Autodesk Inventor part; units mm, degrees
ref_plane "YZ Plane" through (0, 0, 0) normal (1, 0, 0) x (0, 1, 0)
ref_plane "XZ Plane" through (0, 0, 0) normal (0, 1, 0) x (-1, 0, 0)
ref_plane "XY Plane" through (0, 0, 0) normal (0, 0, 1) x (1, 0, 0)
sketch "Sketch1" plane through (0, 0, 0) normal (0, 1, 0) x (-1, 0, 0)
  line L0 (0, 0) -> (-269.875, 0)
  line L1 (-269.875, 0) -> (-269.875, -157.1625)
  line L2 (-269.875, -157.1625) -> (0, -157.1625)
  line L3 (0, -157.1625) -> (0, 0)
  circle A0 centre (-257.175, -148.2725) radius 2.7559
  circle A1 centre (-257.175, -8.89) radius 2.7559
  circle A2 centre (-12.7, -8.89) radius 2.7559
  circle A3 centre (-257.175, -131.1275) radius 2.7559
  circle A4 centre (-257.175, -26.035) radius 2.7559
  circle A5 centre (-12.7, -148.2725) radius 2.7559
  circle A6 centre (-12.7, -131.1275) radius 2.7559
  circle A7 centre (-12.7, -26.035) radius 2.7559
  circle A8 centre (-244.475, -62.5475) radius 4.6609
  line L4 (-242.5434, -66.7893) -> (-246.4066, -66.7893)
  line L5 (-254, -66.7893) -> (-254, -58.3057) construction
  line L6 (-246.4066, -58.3057) -> (-242.5434, -58.3057)
  line L7 (-236.5375, -58.3057) -> (-236.5375, -66.7893) construction
  dimension "d0" = 157.1625
  dimension "d1" = 269.875
  dimension "d2" = 12.7
  dimension "d3" = 8.89
  dimension "d6" = 8.89
  dimension "d7" = 12.7
  dimension "d8" = 12.7
  dimension "d9" = 8.89
  dimension "d11" = 5.5118
  dimension "d12" = 5.5118
  dimension "d13" = 5.5118
  dimension "d15" = 17.145
  dimension "d16" = 12.7
  dimension "d17" = 5.5118
  dimension "d18" = 5.5118
  dimension "d19" = 12.7
  dimension "d20" = 17.145
  dimension "d21" = 12.7
  dimension "d22" = 8.89
  dimension "d23" = 5.5118
  dimension "d24" = 17.145
  dimension "d25" = 12.7
  dimension "d26" = 5.5118
  dimension "d27" = 12.7
  dimension "d28" = 17.145
  dimension "d29" = 5.5118
  dimension "d32" = 25.4
  dimension "d33" = 9.3218
  dimension "d34" = 4.2418
  dimension "d35" = 4.2418
  dimension "d36" = 17.4625
  dimension "d37" = 15.875
  dimension "d38" = 94.615
extrude "Extrusion2" add sketch "Sketch1" along normal blind 5.7658 contours L3 L2 L1 L0 | L6 A8 | A8 L4
properties part number "2023 1 17 Computer Box Door" material "Polycarbonate, Clear"
Check sheet for the modelled part. Datum: model origin and axes. Units: mm. A direction names the side the tool comes from. Coordinates: 2 decimals unless noted, no trailing zeros. Loops run counter-clockwise (first coordinate to the right, second up) from the corner with the lowest first, then second, coordinate; pieces in that order, holes last. Notation, with made-up numbers: (5.5, 23) -> (41.5, 23) arc R22 cw to (41.5, 47) -> close; hole circle Ø6 at (39, 53.5). An arc over 180 degrees is marked (long way). Write item = value, one per line. Start each with the question number.
1. Tool access check on faces 1 (the flat face through (137, 0, -77)), 2 (the cylindrical face through (239.815, 2.843, -62.473)). Record the directions out of +Z, -Z, +X, -X, +Y, -Y that give a thin tool (end or side, any length) a straight path to the whole face; none if there is none.
2. Draft check along X on faces 3 (the cylindrical face through (13.059, 2.843, -11.622)), 4 (the flat face through (269.875, 3, -77)), 5 (the flat face through (137, 5.766, -77)). Enter one of: released by +X, released by -X, zero draft, split by the parting line, or undercut.
3. Section check A-A on x = 12.7. Record the cut outline in (y, z).
4. Material ranges on line 1 (Z direction, x = 12.7, y = 3.15), recorded low to high.
5. Section check B-B on z = -8.89. Record the cut outline in (x, y) (3 decimals), then the cut area to 3 significant figures.
Responses:
q1.face_1 = +Z, -Z, +X, -X, -Y
q1.face_2 = +Y, -Y
q2.face_3 = undercut
q2.face_4 = released by +X
q2.face_5 = zero draft
q3.outline = (0, -157.16) -> (5.77, -157.16) -> (5.77, -151.03) -> (0, -151.03) -> close; (0, -145.52) -> (5.77, -145.52) -> (5.77, -133.88) -> (0, -133.88) -> close; (0, -128.37) -> (5.77, -128.37) -> (5.77, -28.79) -> (0, -28.79) -> close; (0, -23.28) -> (5.77, -23.28) -> (5.77, -11.65) -> (0, -11.65) -> close; (0, -6.13) -> (5.77, -6.13) -> (5.77, 0) -> (0, 0) -> close
q4.line_1 = -157.16 to -151.03, -145.52 to -133.88, -128.37 to -28.79, -23.28 to -11.65, -6.13 to 0
q5.outline = (0, 0) -> (9.944, 0) -> (9.944, 5.766) -> (0, 5.766) -> close; (15.456, 0) -> (254.419, 0) -> (254.419, 5.766) -> (15.456, 5.766) -> close; (259.931, 0) -> (269.875, 0) -> (269.875, 5.766) -> (259.931, 5.766) -> close
q5.area = 1,490 mm2
